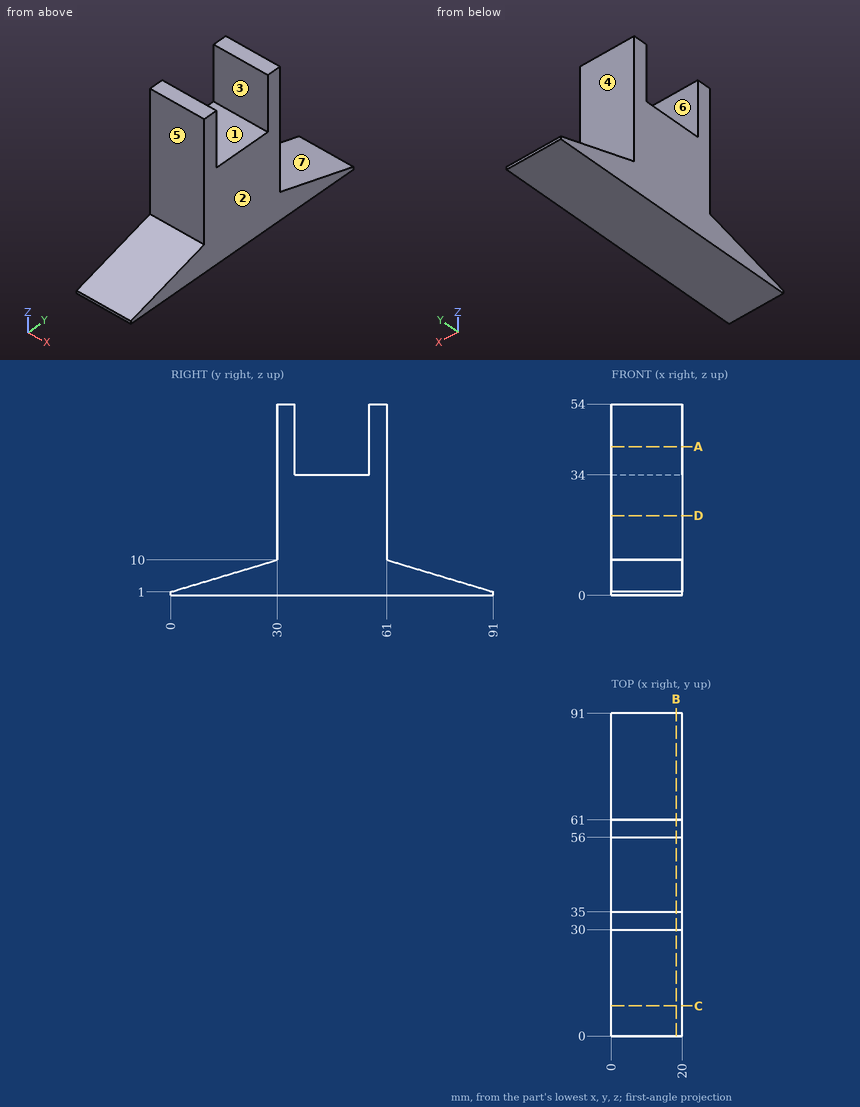
Part print with two shaded views. Sizes in mm from the minimum x, y, z corner. A direction names the side the tool comes from. Round coordinates to 2 decimals unless told otherwise and drop trailing zeros. Order: outer loops, then holes, each group sorted by start corner. A loop starts at its lowest first (then second) coordinate and runs counter-clockwise, first axis right, second up.
(1) Drill centre lines: line 1 (Y direction, x = 4.75, z = 39.5); line 2 (Y direction, x = 3, z = 23.5); line 3 (Z direction, x = 12.25, y = 53). Where is each one in solid material? Low to high.
(2) 3-axis set-ups, long thin cutter, end or side, ignore diameter. For the marked faces 5, 6 and 7: which of +Z, -Z, +X, -X, +Y, -Y reach the whole face in a straight line?
(3) Band-saw the part on A-A (z = 42). List the corners of the cut face in (x, y).
(4) Band-saw the part on D-D (z = 22.5). List the corners of the cut face in (x, y).
(5) Band-saw the part on C-C (y = 8.5). List the corners of the cut face in (x, z), then the cut area to 3 significant figures.
(6) Pin check, flat tips, straight feed: pin 1 (10 mm diameter, centred on x = 8.5, z = 29.5, fed in from -Y); pin 2 (3 mm diameter, centred on x = 16.5, y = 26, fed in from +Z); pin 3 (10 mm diameter, centred on x = 6.5, z = 33, fed in from +Y). Stop position of each tip, or through.
(7) Band-saw the part on B-B (x = 18.25). List the corners of the cut face in (y, z), then the cut area to 3 significant figures.
(8) Pull direction Y, two halves, no side cores. Call the marked faces 1, 2, 3 and 4: released by +Y, released by -Y, zero draft, split by the parting line, or undercut.
Verdict:
1. line 1: y = 30 to 35, 56 to 61
1. line 2: y = 30 to 61
1. line 3: z = 0 to 34
2. face 5: +Z, +X, -X, -Y
2. face 6: +Z, +X, -X
2. face 7: +Z, +X, -X, +Y
3. outline: (0, 30) - (20, 30) - (20, 35) - (0, 35) - close; (0, 56) - (20, 56) - (20, 61) - (0, 61) - close
4. outline: (0, 30) - (20, 30) - (20, 61) - (0, 61) - close
5. outline: (0, 0) - (20, 0) - (20, 3.55) - (0, 3.55) - close
5. area: 71.0 mm2
6. pin 1: stops at y = 30
6. pin 2: stops at z = 9.25
6. pin 3: stops at y = 61
7. outline: (0, 0) - (91, 0) - (91, 1) - (61, 10) - (61, 54) - (56, 54) - (56, 34) - (35, 34) - (35, 54) - (30, 54) - (30, 10) - (0, 1) - close
7. area: 1,580 mm2
8. face 1: undercut
8. face 2: zero draft
8. face 3: undercut
8. face 4: released by +Y
